Model file for the job. Use its own axes, mm. Coordinates: 2 decimals unless noted, no trailing zeros. Write each loop counter-clockwise with the first axis right and the second up, starting at its lowest first coordinate (ties: lowest second). Pieces come first, ordered by that corner, then holes. Notation, with made-up numbers: (87.5, -33) -> (142.5, -33) arc R10 ccw to (142.5, -29) -> close; hole circle Ø1 at (74, 55.25). An arc over 180 degrees is marked (long way). Answer as a JSON object with one key per item and string values. Group by question number.
from build123d import *

# Parameters (mm, degrees)
SKETCH1_W                            = 155
SKETCH1_H                            = 280
BOSS_EXTRUDE1_DEPTH                  = 1.143
M5_CLEARANCE_HOLE1_D                 = 5.5
TOP_SIDE_M3_FLAT_HEAD_AT_2_COUNT     = 2
TOP_SIDE_M3_FLAT_HEAD_AT_2_PITCH     = 85
TOP_SIDE_M3_FLAT_HEAD_AT_3_COUNT     = 2
TOP_SIDE_M3_FLAT_HEAD_AT_3_PITCH     = 87.982327771
TOP_SIDE_M3_FLAT_HEAD_AT_4_COUNT     = 2
TOP_SIDE_M3_FLAT_HEAD_AT_4_PITCH     = 118.226435284
TOP_SIDE_M3_FLAT_HEAD_AT_5_COUNT     = 2
TOP_SIDE_M3_FLAT_HEAD_AT_5_PITCH     = 70.044628631
TOP_SIDE_M3_FLAT_HEAD_AT_6_COUNT     = 2
TOP_SIDE_M3_FLAT_HEAD_AT_6_PITCH     = 129.661598016
TOP_SIDE_M3_FLAT_HEAD_AT_7_COUNT     = 2
TOP_SIDE_M3_FLAT_HEAD_AT_7_PITCH     = 129.743653506
TOP_SIDE_M3_FLAT_HEAD_AT_8_COUNT     = 2
TOP_SIDE_M3_FLAT_HEAD_AT_8_PITCH     = 70.419568481
TOP_SIDE_M3_FLAT_HEAD_AT_9_COUNT     = 2
TOP_SIDE_M3_FLAT_HEAD_AT_9_PITCH     = 99.622365084
TOP_SIDE_M3_FLAT_HEAD_AT_10_COUNT    = 2
TOP_SIDE_M3_FLAT_HEAD_AT_10_PITCH    = 108.939045457
ROUTER_M3_MOUNTING_D                 = 7.4
CUT_EXTRUDE1_REACH                   = 162.036
SKETCH10_W                           = 22.5
SKETCH10_H                           = 50
FILLET1_R                            = 10
POWER_TERMINAL_BLOCKS_M2_5_INSERTS_D = 4.4
M3_GROUNDING_WIRE_HOLE_D             = 3.4
CUT_EXTRUDE2_START                   = -2.286
CUT_EXTRUDE2_DEPTH                   = 2.286
CUT_EXTRUDE3_REACH                   = 162.036
SKETCH17_R                           = 3.25


with BuildPart() as part:
    # Sketch1 → Boss-Extrude1 (new, symmetric)
    with BuildSketch(Plane(origin=(0, 0, 0), x_dir=(1, 0, 0), z_dir=(0, 1, 0))):
        Rectangle(SKETCH1_W, SKETCH1_H)
    extrude(amount=BOSS_EXTRUDE1_DEPTH, both=True)

    # M5 Clearance Hole1 (through all)
    with Locations(Plane(origin=(0, 1.143, 0), x_dir=(1, 0, 0), z_dir=(0, 1, 0))):
        with Locations((47.5, -125), (-47.5, 125), (-47.5, -125), (47.5, 125), (67, 15), (-67, 15)):
            Hole(M5_CLEARANCE_HOLE1_D / 2)

    # Sketch7 → Top Side M3 Flat Head (revolve, cut)
    with BuildSketch(Plane(origin=(42.5, -1.143, -15), x_dir=(0, 0, -1), z_dir=(1, 0, 0))):
        Polygon((0, 0), (0, 2.286), (1.7, 2.286), (1.7, 1.45), (3.15, 0), align=None)
    top_side_m3_flat_head = revolve(axis=Axis((42.5, -7.493, -15), (0, 1, 0)), mode=Mode.SUBTRACT)

    # Top Side M3 Flat Head at 2: Top Side M3 Flat Head ×2
    with Locations(*[(-i * TOP_SIDE_M3_FLAT_HEAD_AT_2_PITCH, 0, 0) for i in range(1, TOP_SIDE_M3_FLAT_HEAD_AT_2_COUNT)]):
        add(top_side_m3_flat_head, mode=Mode.SUBTRACT)

    # Top Side M3 Flat Head at 3: Top Side M3 Flat Head ×2
    with Locations(*[Vector(-0.6058034761110396, 0, 0.7956143213465814) * (i * TOP_SIDE_M3_FLAT_HEAD_AT_3_PITCH) for i in range(1, TOP_SIDE_M3_FLAT_HEAD_AT_3_COUNT)]):
        add(top_side_m3_flat_head, mode=Mode.SUBTRACT)

    # Top Side M3 Flat Head at 4: Top Side M3 Flat Head ×2
    with Locations(*[Vector(-0.021145862970418993, 0, 0.9997764012414158) * (i * TOP_SIDE_M3_FLAT_HEAD_AT_4_PITCH) for i in range(1, TOP_SIDE_M3_FLAT_HEAD_AT_4_COUNT)]):
        add(top_side_m3_flat_head, mode=Mode.SUBTRACT)

    # Top Side M3 Flat Head at 5: Top Side M3 Flat Head ×2
    with Locations(*[Vector(-0.035691530512412285, 0, 0.9993628543475496) * (i * TOP_SIDE_M3_FLAT_HEAD_AT_5_PITCH) for i in range(1, TOP_SIDE_M3_FLAT_HEAD_AT_5_COUNT)]):
        add(top_side_m3_flat_head, mode=Mode.SUBTRACT)

    # Top Side M3 Flat Head at 6: Top Side M3 Flat Head ×2
    with Locations(*[Vector(-0.4110700532436934, 0, 0.9116037578499921) * (i * TOP_SIDE_M3_FLAT_HEAD_AT_6_PITCH) for i in range(1, TOP_SIDE_M3_FLAT_HEAD_AT_6_COUNT)]):
        add(top_side_m3_flat_head, mode=Mode.SUBTRACT)

    # Top Side M3 Flat Head at 7: Top Side M3 Flat Head ×2
    with Locations(*[Vector(-0.6408020566213286, 0, -0.7677061444523389) * (i * TOP_SIDE_M3_FLAT_HEAD_AT_7_PITCH) for i in range(1, TOP_SIDE_M3_FLAT_HEAD_AT_7_COUNT)]):
        add(top_side_m3_flat_head, mode=Mode.SUBTRACT)

    # Top Side M3 Flat Head at 8: Top Side M3 Flat Head ×2
    with Locations(*[Vector(-0.026413112720383172, 0, -0.999651112877098) * (i * TOP_SIDE_M3_FLAT_HEAD_AT_8_PITCH) for i in range(1, TOP_SIDE_M3_FLAT_HEAD_AT_8_COUNT)]):
        add(top_side_m3_flat_head, mode=Mode.SUBTRACT)

    # Top Side M3 Flat Head at 9: Top Side M3 Flat Head ×2
    with Locations(*[Vector(-0.01867050635090894, 0, -0.9998256909044699) * (i * TOP_SIDE_M3_FLAT_HEAD_AT_9_PITCH) for i in range(1, TOP_SIDE_M3_FLAT_HEAD_AT_9_COUNT)]):
        add(top_side_m3_flat_head, mode=Mode.SUBTRACT)

    # Top Side M3 Flat Head at 10: Top Side M3 Flat Head ×2
    with Locations(*[Vector(-0.763179075523523, 0, -0.6461870462049366) * (i * TOP_SIDE_M3_FLAT_HEAD_AT_10_PITCH) for i in range(1, TOP_SIDE_M3_FLAT_HEAD_AT_10_COUNT)]):
        add(top_side_m3_flat_head, mode=Mode.SUBTRACT)

    # Router M3 Mounting (through all)
    with Locations(Plane(origin=(0, 1.143, 0), x_dir=(1, 0, 0), z_dir=(0, 1, 0))):
        with Locations((-23.5, -75.5), (-23.5, 103.5), (51.5, -4)):
            Hole(ROUTER_M3_MOUNTING_D / 2)

    # Sketch10 → Cut-Extrude1 (cut, up to next)
    with BuildSketch(Plane(origin=(0, 1.143, 0), x_dir=(1, 0, 0), z_dir=(0, 1, 0)), mode=Mode.PRIVATE) as cut_extrude1_sk1:
        with Locations((-66.25, 115)):
            Rectangle(SKETCH10_W, SKETCH10_H)
    cut_extrude1_tool1 = extrude(cut_extrude1_sk1.sketch, amount=-CUT_EXTRUDE1_REACH, mode=Mode.PRIVATE) & part.part
    # Sketch10 → Cut-Extrude1 (cut, up to next)
    with BuildSketch(Plane(origin=(0, 1.143, 0), x_dir=(1, 0, 0), z_dir=(0, 1, 0)), mode=Mode.PRIVATE) as cut_extrude1_sk2:
        with Locations((66.25, 115)):
            Rectangle(SKETCH10_W, SKETCH10_H)
    cut_extrude1_tool2 = extrude(cut_extrude1_sk2.sketch, amount=-CUT_EXTRUDE1_REACH, mode=Mode.PRIVATE) & part.part
    add(cut_extrude1_tool1.solids().sort_by_distance((-66.25, 1.143, -115))[0], mode=Mode.SUBTRACT)
    add(cut_extrude1_tool2.solids().sort_by_distance((66.25, 1.143, -115))[0], mode=Mode.SUBTRACT)

    # Fillet1
    fillet1_edges = [part.edges().sort_by_distance(p)[0] for p in [
        (-77.5, 0, -90),
        (-55, 0, -140),
        (-55, 0, -90),
        (77.5, 0, -90),
        (55, 0, -90),
        (55, 0, -140),
        (77.5, 0, 140),
        (-77.5, 0, 140),
    ]]
    fillet(fillet1_edges, radius=FILLET1_R)

    # Power Terminal Blocks M2.5 Inserts (through all)
    with Locations(Plane(origin=(0, 1.143, 0), x_dir=(1, 0, 0), z_dir=(0, 1, 0))):
        with Locations((-65, -112), (-65, -54)):
            Hole(POWER_TERMINAL_BLOCKS_M2_5_INSERTS_D / 2)

    # M3 grounding wire hole (through all)
    with Locations(Plane(origin=(0, 1.143, 0), x_dir=(1, 0, 0), z_dir=(0, 1, 0))):
        with Locations((-67.5, -130)):
            Hole(M3_GROUNDING_WIRE_HOLE_D / 2)

    # Sketch15 → Cut-Extrude2 (cut)
    with BuildSketch(Plane(origin=(0, 1.143, 0), x_dir=(1, 0, 0), z_dir=(0, 1, 0)).offset(CUT_EXTRUDE2_START)):
        with BuildLine():
            Line((44.75, 124.5), (44.75, 125.5))
            ThreePointArc((44.75, 125.5), (47.5, 128.25), (50.25, 125.5))
            Line((50.25, 125.5), (50.25, 124.5))
            ThreePointArc((50.25, 124.5), (47.5, 121.75), (44.75, 124.5))
        make_face()
        with BuildLine():
            Line((-44.75, 125.5), (-44.75, 124.5))
            ThreePointArc((-44.75, 124.5), (-47.5, 121.75), (-50.25, 124.5))
            Line((-50.25, 124.5), (-50.25, 125.5))
            ThreePointArc((-50.25, 125.5), (-47.5, 128.25), (-44.75, 125.5))
        make_face()
        with BuildLine():
            Line((-44.75, -124.5), (-44.75, -125.5))
            ThreePointArc((-44.75, -125.5), (-47.5, -128.25), (-50.25, -125.5))
            Line((-50.25, -125.5), (-50.25, -124.5))
            ThreePointArc((-50.25, -124.5), (-47.5, -121.75), (-44.75, -124.5))
        make_face()
        with BuildLine():
            Line((50.25, -124.5), (50.25, -125.5))
            ThreePointArc((50.25, -125.5), (47.5, -128.25), (44.75, -125.5))
            Line((44.75, -125.5), (44.75, -124.5))
            ThreePointArc((44.75, -124.5), (47.5, -121.75), (50.25, -124.5))
        make_face()
    extrude(amount=CUT_EXTRUDE2_DEPTH, mode=Mode.SUBTRACT)

    # Sketch17 → Cut-Extrude3 (cut, up to next)
    with BuildSketch(Plane(origin=(0, 1.143, 0), x_dir=(1, 0, 0), z_dir=(0, 1, 0)), mode=Mode.PRIVATE) as cut_extrude3_sk1:
        with Locations(Location((-67, 32.75, 0), (0, 0, 270))):
            Circle(SKETCH17_R)
    cut_extrude3_tool1 = extrude(cut_extrude3_sk1.sketch, amount=-CUT_EXTRUDE3_REACH, mode=Mode.PRIVATE) & part.part
    # Sketch17 → Cut-Extrude3 (cut, up to next)
    with BuildSketch(Plane(origin=(0, 1.143, 0), x_dir=(1, 0, 0), z_dir=(0, 1, 0)), mode=Mode.PRIVATE) as cut_extrude3_sk2:
        with Locations(Location((-67, 46.833333333, 0), (0, 0, 270))):
            Circle(SKETCH17_R)
    cut_extrude3_tool2 = extrude(cut_extrude3_sk2.sketch, amount=-CUT_EXTRUDE3_REACH, mode=Mode.PRIVATE) & part.part
    # Sketch17 → Cut-Extrude3 (cut, up to next)
    with BuildSketch(Plane(origin=(0, 1.143, 0), x_dir=(1, 0, 0), z_dir=(0, 1, 0)), mode=Mode.PRIVATE) as cut_extrude3_sk3:
        with Locations(Location((-67, 60.916666667, 0), (0, 0, 270))):
            Circle(SKETCH17_R)
    cut_extrude3_tool3 = extrude(cut_extrude3_sk3.sketch, amount=-CUT_EXTRUDE3_REACH, mode=Mode.PRIVATE) & part.part
    # Sketch17 → Cut-Extrude3 (cut, up to next)
    with BuildSketch(Plane(origin=(0, 1.143, 0), x_dir=(1, 0, 0), z_dir=(0, 1, 0)), mode=Mode.PRIVATE) as cut_extrude3_sk4:
        with Locations(Location((-67, 75, 0), (0, 0, 270))):
            Circle(SKETCH17_R)
    cut_extrude3_tool4 = extrude(cut_extrude3_sk4.sketch, amount=-CUT_EXTRUDE3_REACH, mode=Mode.PRIVATE) & part.part
    add(cut_extrude3_tool1.solids().sort_by_distance((-67, 1.143, -32.75))[0], mode=Mode.SUBTRACT)
    add(cut_extrude3_tool2.solids().sort_by_distance((-67, 1.143, -46.833333))[0], mode=Mode.SUBTRACT)
    add(cut_extrude3_tool3.solids().sort_by_distance((-67, 1.143, -60.916667))[0], mode=Mode.SUBTRACT)
    add(cut_extrude3_tool4.solids().sort_by_distance((-67, 1.143, -75))[0], mode=Mode.SUBTRACT)


solid = part.part
(1) Cut at B-B on y = 0.8. Give the number of separate pieces and of enclosed holes in the cut face, plus the area to 3 significant figures.
(2) Pin check, flat tips, straight feed: pin 1 (4 mm diameter, centred on x = -65, z = 112, fed in from -Y); pin 2 (5.5 mm diameter, centred on x = -10.8, z = 103.2, fed in from +Y); pin 3 (5.5 mm diameter, centred on x = -42.5, z = -15, fed in from -Y); pin 4 (0.7 mm diameter, centred on y = 0, z = -119, fed in from -X). Stop position of each tip, or through.
(3) Cut at A-A on z = 4. List the corners of the cut face in (x, y), plus the area to 3 significant figures.
(4) Pull direction X, two halves, no side cores. Call faces 1 (the face through (-66.86, 0.02, -50.08)), 2 (the face through (57.85, -0.02, -93.01)), 3 (the face through (-74.65, -0.02, -86.99)): released by +X, released by -X, zero draft, split by the parting line, or undercut.
(5) Wall check: probe 1 along Z at (x, y) = (-23.5, 0.7); probe 2 along X at (y, z) = (0.55, -15); probe 3 along Z at (x, y) = (37.5, -0.9). Give the ranges that are in metal, low to high.
Results found:
{
 "1": {"separate pieces": "1", "enclosed holes": "26", "area": "40,500 mm²"},
 "2": {"pin 1": "passes through", "pin 2": "stops at y = 1.14", "pin 3": "stops at y = -0.74", "pin 4": "stops at x = -55"},
 "3": {"outline": "(-77.5, -1.14) -> (47.8, -1.14) -> (47.8, 1.14) -> (-77.5, 1.14) -> close; (55.2, -1.14) -> (77.5, -1.14) -> (77.5, 1.14) -> (55.2, 1.14) -> close", "area": "337 mm²"},
 "4": {"face 1": "undercut", "face 2": "released by +X", "face 3": "released by -X"},
 "5": {"probe 1": "z = -140 to -107.2, -99.8 to 71.8, 79.2 to 140", "probe 2": "x = -77.5 to -69.75, -64.25 to -44.2, -40.8 to 40.8, 44.2 to 64.25, 69.75 to 77.5", "probe 3": "z = -140 to 53.52, 56.48 to 101.72, 104.68 to 140"}
}
